Model file for the job. Use its own axes, mm. A direction names the side the tool comes from. Coordinates: 2 decimals unless noted, no trailing zeros. Order: outer loops, then holes, each group sorted by start corner. A loop starts at its lowest first (then second) coordinate and runs counter-clockwise, first axis right, second up. Notation, with made-up numbers: M 6,88 L 37,88 A19 cw 37,107 Z; hole C 14.5,26 d2. An arc over 180 degrees is marked long. Return JSON: item names as keys, results as strings.
Autodesk Inventor part; units mm, degrees
ref_plane "YZ Plane" through (0, 0, 0) normal (1, 0, 0) x (0, 1, 0)
ref_plane "XZ Plane" through (0, 0, 0) normal (0, 1, 0) x (-1, 0, 0)
ref_plane "XY Plane" through (0, 0, 0) normal (0, 0, 1) x (1, 0, 0)
sketch "Skizze1" plane through (0, 0, 0) normal (0, 1, 0) x (-1, 0, 0)
  line L0 (40, -3.5) -> (-40, -3.5)
  line L1 (-40, -3.5) -> (-40, 3.5)
  line L2 (-40, 3.5) -> (-30, 3.5)
  line L3 (40, 3.5) -> (40, -3.5)
  line L4 (40, -3.5) -> (-40, 3.5) construction
  line L5 (-40, -3.5) -> (40, 3.5) construction
  line L6 (40, 3.5) -> (30, 3.5)
  line L7 (30, 3.5) -> (30, 18.5)
  line L8 (30, 18.5) -> (40, 18.5)
  line L9 (40, 18.5) -> (40, 3.5)
  circle A0 centre (35, 11.5) radius 3
  line L10 (0, 43.2114) -> (0, -35.1785) construction
  line L11 (-30, 3.5) -> (-30, 18.5)
  line L12 (-30, 18.5) -> (-40, 18.5)
  line L13 (-40, 18.5) -> (-40, 3.5)
  circle A1 centre (-35, 11.5) radius 3
  line L14 (-30, 3.5) -> (30, 3.5)
  line L15 (30, 3.5) -> (40, 3.5)
  line L16 (30, 3.5) -> (30, -3.5)
  line L17 (-30, 3.5) -> (-30, -3.5)
  point P0 (0, 0)
  point P1 (30, 11)
  dimension "d0" = 80
  dimension "d1" = 7
  dimension "d4" = 10
  dimension "d5" = 15
  dimension "d6" = 6
  dimension "d7" = 7
  dimension "d8" = 5
extrude "Extrusion1" add sketch "Skizze1" along normal blind 60 contours L0 L16 L6 L3 | L0 L17 L14 L16 | L0 L1 L2 L17
extrude "Extrusion2" add sketch "Skizze1" along normal blind 5 contours L6 L7 L8 L9 | L2 L13 L12 L11
extrude "Extrusion3" cut sketch "Skizze1" along normal blind 21 contours L0 L17 L14 L16
sketch "Skizze2" plane through (-40, 60, 3.5) normal (0, 0, 1) x (1, 0, 0)
  line L0 (40, -60) -> (40, 40) construction
  circle A0 centre (32, -4.5) radius 2
  line L1 (70, -60) -> (80, -60)
  line L2 (40, -12.5) -> (0, -12.5) construction
  line L3 (0, -55) -> (0, 0) construction
  circle A1 centre (48, -4.5) radius 2
  circle A2 centre (32, -20.5) radius 2
  circle A3 centre (48, -20.5) radius 2
  circle A4 centre (40, -12.5) radius 6
  line L4 (0, 0) -> (80, 0)
  line L5 (27.5, -25) -> (52.5, -25)
  line L6 (52.5, -25) -> (52.5, 0)
  line L7 (52.5, 0) -> (27.5, 0)
  line L8 (27.5, 0) -> (27.5, -25)
  line L9 (27.5, -25) -> (52.5, 0) construction
  line L10 (52.5, -25) -> (27.5, 0) construction
  line L11 (27.5, -25) -> (0, -25)
  line L12 (0, -25) -> (0, 0)
  line L13 (0, 0) -> (27.5, 0)
  line L14 (27.5, 0) -> (27.5, -25)
  line L15 (80, -55) -> (80, 0)
  line L16 (52.5, -25) -> (80, -25)
  line L17 (80, -25) -> (80, 0)
  line L18 (80, 0) -> (52.5, 0)
  line L19 (52.5, 0) -> (52.5, -25)
  dimension "d14" = 4
  dimension "d15" = 47.5
  dimension "d16" = 8
  dimension "d17" = 8
  dimension "d20" = 16
  dimension "d23" = 16
  dimension "d26" = 12
  dimension "d27" = 25
extrude "Extrusion4" cut sketch "Skizze2" against normal up to surface (7 mm away) contours A0 | A1 | A2 | A3 | A4 | L4 L8 L11 L12 | L4 L15 L16 L6
fillet "Rundung1" radius 5 8 edges at (-40, 35, 0) (-12.5, 35, 0) (-12.5, 60, 0) (12.5, 60, 0) (12.5, 35, 0) (40, 35, 0) (-35, 0, -3.5) (35, 0, -3.5)
properties part number "Bracket vorne"
Item 1: Saw through at D-D (z = -1.25). Write the cut outline in (x, y).
Check result:
{"outline": "M -40,0.82 L -30,0.82 L -30,21 L 30,21 L 30,0.82 L 40,0.82 L 40,30 A5 ccw 35,35 L 17.5,35 A5 cw 12.5,40 L 12.5,55 A5 ccw 7.5,60 L -7.5,60 A5 ccw -12.5,55 L -12.5,40 A5 cw -17.5,35 L -35,35 A5 ccw -40,30 Z; hole C -8,39.5 d4; hole C -8,55.5 d4; hole C 0,47.5 d12; hole C 8,39.5 d4; hole C 8,55.5 d4"}
Item 2: Saw through at B-B (y = 47.5). Write the cut outline in (x, z), and give its area (3 significant figures).
Check result:
{"outline": "M -12.5,-3.5 L -6,-3.5 L -6,3.5 L -12.5,3.5 Z; M 6,-3.5 L 12.5,-3.5 L 12.5,3.5 L 6,3.5 Z", "area": "91.0 mm2"}
Item 3: 3-axis set-ups, long thin cutter, end or side, ignore diameter. For faces 1 (the flat face through (-26, 35, 0)), 2 (the cylindrical face through (7.566, 37.548, 0.049)), 3 (the flat face through (30, 8, 3)), 4 (the flat face through (37, 5, 9)), 5 (the flat face through (26, 35, 0)): which of +Z, -Z, +X, -X, +Y, -Y reach the whole face in a straight line?
Check result:
{"face 1": "+Z, -Z, -X, +Y", "face 2": "+Z, -Z", "face 3": "+Z, -Z, -Y", "face 4": "+Z, +X, -X, +Y", "face 5": "+Z, -Z, +X, +Y"}
Item 4: Saw through at A-A (z = 11.5). Write the cut outline in (x, y), and give its area (3 significant figures).
Check result:
{"outline": "M -40,0 L -38,0 L -38,5 L -40,5 Z; M -32,0 L -30,0 L -30,5 L -32,5 Z; M 30,0 L 32,0 L 32,5 L 30,5 Z; M 38,0 L 40,0 L 40,5 L 38,5 Z", "area": "40.0 mm2"}
Item 5: Pull direction X, two halves, no side cores. Call faces 6 (the flat face through (-1, 32, -3.5)), 7 (the cylindrical face through (-8.434, 37.548, 0.049)), 8 (the cylindrical face through (-39, 33, 0)), 9 (the flat face through (12.5, 47, 0)): +X half, -X half, draft (parallel to the pull), parting line (faces both ways), or undercut.
Check result:
{"face 6": "draft", "face 7": "undercut", "face 8": "-X half", "face 9": "+X half"}
Item 6: Wall check: line 1 (X direction, y = 3.5, z = 8); line 2 (Y direction, x = 8, z = -0.75); line 3 (Z direction, x = -11.5, y = 55.5). Give the ranges that are in metal, low to high.
Check result:
{"line 1": "x = -40 to -30, 30 to 40", "line 2": "y = 21 to 37.5, 41.5 to 53.5, 57.5 to 59.97", "line 3": "z = -3.5 to 3.5"}
Item 7: Saw through at C-C (x = 0). Write the cut outline in (y, z).
Check result:
{"outline": "M 21,-3.5 L 41.5,-3.5 L 41.5,3.5 L 21,3.5 Z; M 53.5,-3.5 L 60,-3.5 L 60,3.5 L 53.5,3.5 Z"}
Item 8: Drop flat-ended pins along their axis: pin 1 Ø7.5 at (x, z) = (14, -0.5) entering from -Y; pin 2 Ø14 at (x, y) = (0, 47.5) entering from +Z; pin 3 Ø12 at (y, z) = (43.5, 2.5) entering from -X. Give the stop position or say it passes through.
Check result:
{"pin 1": "stops at y = 21", "pin 2": "stops at z = 3.5", "pin 3": "stops at x = -13.17"}
